from build123d import *

# Parameters (mm, degrees)
SKETCH1_R           = 13.97
BOSS_EXTRUDE1_DEPTH = 3.175
SKETCH5_R           = 6.35
CUT_EXTRUDE2_DEPTH  = 3.175
CIRPATTERN1_COUNT   = 4


with BuildPart() as part:
    # Sketch1 → Boss-Extrude1 (new body)
    with BuildSketch(Plane(origin=(0, 0, 0), x_dir=(1, 0, 0), z_dir=(0, 1, 0))):
        Circle(SKETCH1_R)
    extrude(amount=BOSS_EXTRUDE1_DEPTH)

    # Sketch5 → Cut-Extrude2 (cut)
    with BuildSketch(Plane(origin=(0, 3.175, 0), x_dir=(1, 0, 0), z_dir=(0, 1, 0))):
        Circle(SKETCH5_R)
    extrude(amount=-CUT_EXTRUDE2_DEPTH, mode=Mode.SUBTRACT)

    # Sketch6 → #4 Clearance Hole1 (revolve, cut)
    with BuildSketch(Plane(origin=(10.16, 3.175, 0), x_dir=(0, 0, 1), z_dir=(1, 0, 0))):
        Polygon((0, 0), (0, 11.140574487), (1.63195, 10.16), (1.63195, 0), align=None)
    f_4_clearance_hole1 = revolve(axis=Axis((10.16, 9.525, 0), (0, -1, 0)), mode=Mode.SUBTRACT)

    # CirPattern1: #4 Clearance Hole1 ×4 about axis
    cirpattern1_axis = Axis((0, 0, 0), (0, 1, 0))
    for i in range(1, CIRPATTERN1_COUNT):
        add(f_4_clearance_hole1.rotate(cirpattern1_axis, i * 360 / CIRPATTERN1_COUNT), mode=Mode.SUBTRACT)


solid = part.part
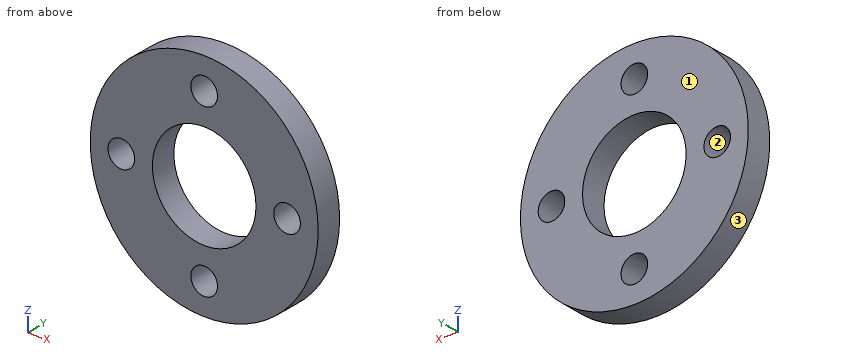
Work out the finished part from the listing and answer in its coordinate system (mm). Face numbers are marked on the shaded views. Round coordinates to 2 decimals unless told otherwise and drop trailing zeros. Write each loop counter-clockwise with the first axis right and the second up, starting at its lowest first coordinate (ties: lowest second). Pieces come first, ordered by that corner, then holes. Notation, with made-up numbers: M 46,71.5 L 75,71.5 A8 ccw 75,82.5 Z; hole C 87.25,-9 d3. An arc over 180 degrees is marked long. Use a Markdown table: item, result.
1) The part is cut by section B-B on z = 0. Give the vertices of the cut face in (x, y) (3 decimals), plus the area to 3 significant figures.
Taken from the geometry:
| item | result |
|---|---|
| outline | M -13.97,0 L -11.792,0 L -11.792,3.175 L -13.97,3.175 Z; M -8.528,0 L -6.35,0 L -6.35,3.175 L -8.528,3.175 Z; M 6.35,0 L 8.528,0 L 8.528,3.175 L 6.35,3.175 Z; M 11.792,0 L 13.97,0 L 13.97,3.175 L 11.792,3.175 Z |
| area | 27.7 mm2 |
2) A flat-ended cylindrical pin translates along its axis: pin 1 (1.5 mm diameter, centred on y = 0.5, z = -5, fed in from -X). Find the tip coordinate at first contact, or state that the pin passes through.
Taken from the geometry:
| item | result |
|---|---|
| pin 1 | stops at x = -13.31 |
3) Determine the mould class of the marked faces 1, 2 and 3 for opening direction Z: pulls with the +Z half, pulls with the -Z half, needs draft (parallel to the pull), parting line crosses it, or undercut.
Taken from the geometry:
| item | result |
|---|---|
| face 1 | needs draft |
| face 2 | undercut |
| face 3 | parting line crosses it |
4) Consider line 1 (Z direction, x = 0, y = 0.85); line 2 (X direction, y = 2.85, z = -1.25). Determine where each line is inside the solid, lowest interval first. Write a range as [from, to].
Taken from the geometry:
| item | result |
|---|---|
| line 1 | z = [-13.97, -11.79], [-8.53, -6.35], [6.35, 8.53], [11.79, 13.97] |
| line 2 | x = [-13.91, -11.21], [-9.11, -6.23], [6.23, 9.11], [11.21, 13.91] |
5) The part is cut by section D-D on z = 10.16. Give the vertices of the cut face in (x, y) (3 decimals), plus the area to 3 significant figures.
Taken from the geometry:
| item | result |
|---|---|
| outline | M -9.588,0 L -1.632,0 L -1.632,3.175 L -9.588,3.175 Z; M 1.632,0 L 9.588,0 L 9.588,3.175 L 1.632,3.175 Z |
| area | 50.5 mm2 |
6) The part is cut by section A-A on x = 0. Give the vertices of the cut face in (y, z) (3 decimals), plus the area to 3 significant figures.
Taken from the geometry:
| item | result |
|---|---|
| outline | M 0,-13.97 L 3.175,-13.97 L 3.175,-11.792 L 0,-11.792 Z; M 0,-8.528 L 3.175,-8.528 L 3.175,-6.35 L 0,-6.35 Z; M 0,6.35 L 3.175,6.35 L 3.175,8.528 L 0,8.528 Z; M 0,11.792 L 3.175,11.792 L 3.175,13.97 L 0,13.97 Z |
| area | 27.7 mm2 |
7) The part is cut by section C-C on y = 1.35. Give the vertices of the cut face in (x, z), plus the area to 3 significant figures.
Taken from the geometry:
| item | result |
|---|---|
| outline | C 0,0 d27.94; hole C -10.16,0 d3.26; hole C 0,0 d12.7; hole C 0,-10.16 d3.26; hole C 0,10.16 d3.26; hole C 10.16,0 d3.26 |
| area | 453 mm2 |
